Verification items for this drawing (mm, ordinates from the low corner). A direction names the side the tool comes from. Round coordinates to 2 decimals unless told otherwise and drop trailing zeros. Order: outer loops, then holes, each group sorted by start corner. A loop starts at its lowest first (then second) coordinate and runs counter-clockwise, first axis right, second up. Notation, with made-up numbers: (-10.5, 26) - (-0.5, 26) arc R24 cw to (-0.5, 59) - close; hole circle Ø10 at (76.25, 31). An arc over 180 degrees is marked (long way). Answer as CSV lines item,"result". Start each with the question number.
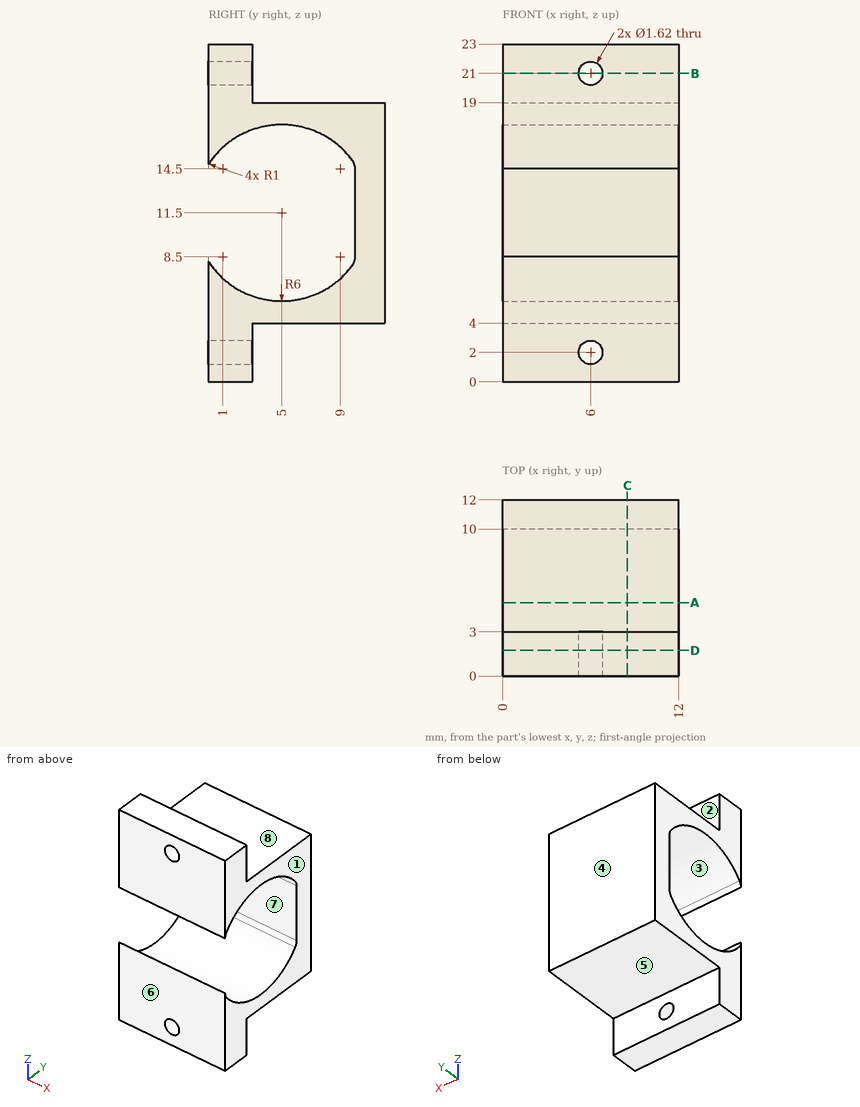
1. Go/stop test with flat-tipped pins: pin 1 Ø1.8 at (x, z) = (5, 12) entering from -Y; pin 2 Ø1.2 at (x, z) = (5.5, 21) entering from +Y. Record where each tip stops, or that it passes through.
2. Section check B-B on z = 21. Record the boundary of the cut face in (x, y).
3. Draft check along Z on the marked faces 6, 7 and 8. Enter one of: released by +Z, released by -Z, zero draft, split by the parting line, or undercut.
4. Thickness scan on probe 1 along Z at (x, y) = (9.25, 5); probe 2 along X at (y, z) = (1.3, 2); probe 3 along Y at (x, z) = (2.5, 9.75). Record the ranges inside material, lowest first.
5. Section check A-A on y = 5. Record the boundary of the cut face in (x, z), plus the area to 3 significant figures.
6. Access from +Z, -Z, +X, -X, +Y, -Y to the whole of each face (thin tool, end or side, straight path). Record for the marked faces 1, 2, 3, 4 and 5.
7. Section check C-C on x = 8.5. Record the boundary of the cut face in (y, z).
8. Section check D-D on y = 1.75. Record the boundary of the cut face in (x, z).
Numbers:
1,pin 1,"stops at y = 10"
1,pin 2,"stops at y = 3"
2,outline,"(0, 0) - (5.19, 0) - (5.19, 3) - (0, 3) - close; (6.81, 0) - (12, 0) - (12, 3) - (6.81, 3) - close"
3,face 6,"zero draft"
3,face 7,"undercut"
3,face 8,"released by +Z"
4,probe 1,"z = 4 to 5.5, 17.5 to 19"
4,probe 2,"x = 0 to 5.19, 6.81 to 12"
4,probe 3,"y = 10 to 12"
5,outline,"(0, 4) - (12, 4) - (12, 5.5) - (0, 5.5) - close; (0, 17.5) - (12, 17.5) - (12, 19) - (0, 19) - close"
5,area,"36.0 mm2"
6,face 1,"+Z, -Z, +X, +Y, -Y"
6,face 2,"+Z, +X, -X, +Y"
6,face 3,"+X, -X"
6,face 4,"+Z, -Z, +X, -X, +Y"
6,face 5,"-Z, +X, -X, +Y"
7,outline,"(0, 0) - (3, 0) - (3, 4) - (12, 4) - (12, 19) - (3, 19) - (3, 23) - (0, 23) - (0, 14.5) arc R1 cw to (0.2, 15.1) arc R6 cw to (9.8, 15.1) arc R1 cw to (10, 14.5) - (10, 8.5) arc R1 cw to (9.8, 7.9) arc R6 cw to (0.2, 7.9) arc R1 cw to (0, 8.5) - close"
8,outline,"(0, 0) - (12, 0) - (12, 6.46) - (0, 6.46) - close; (0, 16.54) - (12, 16.54) - (12, 23) - (0, 23) - close; hole circle Ø1.62 at (6, 2); hole circle Ø1.62 at (6, 21)"
